from build123d import *

# Parameters (mm, degrees)
F1_DEPTH = 25.9842
F2_R     = 12.7
F2_R_2   = 6.35
F3_DEPTH = 25.4
F4_R     = 12.7
F4_R_2   = 6.35
F5_DEPTH = 25.4
F7_R     = 4.860079591
F8_DEPTH = 12.7
F8_TAPER = -7
F6_W     = 22.3425124863
F6_H     = 36.2117751569
F9_DEPTH = 38.6852001


with BuildPart() as f1:
    # F0 (on Top) → F1 (new body)
    with BuildSketch(Plane.XY):
        Polygon((5.17619859, -4.1735334439), (-38.1843136522, -22.134045686), (-12.7843136522, -22.134045686), align=None)
    extrude(amount=F1_DEPTH)

    # F2 (on face) → F3 (join)
    with BuildSketch(Plane(origin=(4.6748660169, -4.6748660169, 0), x_dir=(0.7071067812, 0.7071067812, 0), z_dir=(0.7071067812, -0.7071067812, 0))):
        with Locations((-11.9910086759, 12.9921)):
            Circle(F2_R)
        with Locations((-11.9910086759, 12.9921)):
            Circle(F2_R_2, mode=Mode.SUBTRACT)
    extrude(amount=F3_DEPTH)

    # F4 (on face) → F5 (join)
    with BuildSketch(Plane.XZ.offset(22.134045686)):
        with Locations((-25.4843136522, 12.9921)):
            Circle(F4_R)
        with Locations((-25.4843136522, 12.9921)):
            Circle(F4_R_2, mode=Mode.SUBTRACT)
    extrude(amount=F5_DEPTH)

    # F7 (on face) → F8 (join)
    with BuildSketch(Plane.XY.offset(25.9842)):
        with Locations((-14.6441855916, -17.6439176255)):
            Circle(F7_R)
    extrude(amount=F8_DEPTH, taper=F8_TAPER)

    # F6 (on face) → F9 (cut, through all)
    with BuildSketch(Plane.XY):
        with Locations((-41.7355698953, -31.0400566086)):
            Rectangle(F6_W, F6_H)
        Polygon((34.686883608, -12.8634416315), (9.0812918357, 12.7421501407), (-6.7172502521, -3.0563919471), (18.8883415201, -28.6619837193), align=None)
    extrude(amount=F9_DEPTH, mode=Mode.SUBTRACT)


solid = f1.part
Here's how the part is built. I have some questions about the finished solid (model axes, mm). A direction names the side the tool comes from. Give positions to 0.01 mm unless a question says otherwise; leave off trailing zeros. Order: outer loops, then holes, each group sorted by start corner. A loop starts at its lowest first (then second) coordinate and runs counter-clockwise, first axis right, second up. Notation, with made-up numbers: (70.25, 78) -> (88.25, 78) arc R13 cw to (88.25, 97) -> close; hole circle Ø10 at (-0.75, 17.5). An arc over 180 degrees is marked (long way). Use a Markdown table: item, result. Add a question column.
Item 1: Imagine slicing it at D-D on y = -45. Please give me the cut outline in (x, z).
Item 2: If we mould it in two halves opening along X, with no side actions, what happens to faces 4 (the face through (7.511, -17.285, 18.584)), 5 (the face through (-24, -20, 25.984)), 6 (the face through (-17, -22.134, 3))? For each: pulls with the +X half, pulls with the -X half, needs draft (parallel to the pull), parting line crosses it, or undercut.
Item 3: I need wall thicknesses on line 1 (Z direction, x = -9, y = -12); line 2 (Z direction, x = -26.5, y = -25.5); line 3 (Z direction, x = -1.5, y = -19.5). Which ranges of each line are inside material? Lowest first, please.
Item 4: For faces 1 (the face through (-12.79, -34.66, 12.64)), 2 (the face through (-16.307, -13.072, 12.81)), 3 (the face through (-4.31, -13.66, 12.9)), which set-ups out of +Z, -Z, +X, -X, +Y, -Y let a thin tool reach every point of the face, with its end or its side?
Item 5: Imagine slicing it at C-C on z = 16. Please give me the cut outline in (x, y), plus the area to 3 significant figures.
Item 6: Imagine slicing it at B-B on x = -25.5. Please give me the cut outline in (y, z).
Item 7: Imagine slicing it at A-A on z = 8. Please give me the cut outline in (x, y).
Item 8: Will these pins go through, and if not, where does the flat tip stop? pin 1 (1.5 mm diameter, centred on x = -17, z = 26, fed in from +Y); pin 2 (20.5 mm diameter, centred on x = -25.48, z = 12.99, fed in from +Y); pin 3 (6 mm diameter, centred on x = 12.5, y = -17, fed in from +Z); pin 4 (3.5 mm diameter, centred on x = -25, z = 13, fed in from -Y).
Data:
| question | item | result |
|---|---|---|
| 1 | outline | (-30.56, 1.35) arc R12.7 ccw (long way) to (-30.56, 24.63) -> (-30.56, 16.8) arc R6.35 cw (long way) to (-30.56, 9.18) -> close |
| 2 | face 4 | pulls with the +X half |
| 2 | face 5 | needs draft |
| 2 | face 6 | undercut |
| 3 | line 1 | z = 0 to 25.98 |
| 3 | line 2 | z = 0.33 to 6.72, 19.26 to 25.65 |
| 3 | line 3 | z = 0.62 to 7.32, 18.66 to 25.37 |
| 4 | face 1 | -Y |
| 4 | face 2 | -Z, -X, +Y |
| 4 | face 3 | none |
| 5 | outline | (-30.56, -22.13) -> (-19.89, -22.13) -> (-19.89, -47.53) -> (-13.15, -47.53) -> (-13.15, -22.13) -> (-12.78, -22.13) -> (-12.53, -21.88) -> (5.43, -39.84) -> (10.2, -35.07) -> (-7.76, -17.11) -> (-0.21, -9.56) -> (-2.44, -7.33) -> (-30.56, -18.98) -> close |
| 5 | area | 547 mm² |
| 6 | outline | (-47.53, 0.29) -> (-22.13, 0.29) -> (-22.13, 0) -> (-16.88, 0) -> (-16.88, 25.98) -> (-22.13, 25.98) -> (-22.13, 25.69) -> (-47.53, 25.69) -> (-47.53, 19.34) -> (-22.13, 19.34) -> (-22.13, 6.64) -> (-47.53, 6.64) -> close |
| 7 | outline | (-30.56, -47.53) -> (-29.41, -47.53) -> (-29.41, -22.13) -> (-21.56, -22.13) -> (-21.56, -47.53) -> (-13.81, -47.53) -> (-13.81, -22.13) -> (-12.78, -22.13) -> (-12.06, -21.41) -> (5.9, -39.37) -> (11.38, -33.89) -> (-6.58, -15.93) -> (-1.03, -10.38) -> (16.93, -28.34) -> (17.75, -27.52) -> (-2.44, -7.33) -> (-30.56, -18.98) -> close |
| 8 | pin 1 | stops at y = -13.04 |
| 8 | pin 2 | stops at y = -12.63 |
| 8 | pin 3 | passes through |
| 8 | pin 4 | stops at y = -22.13 |
